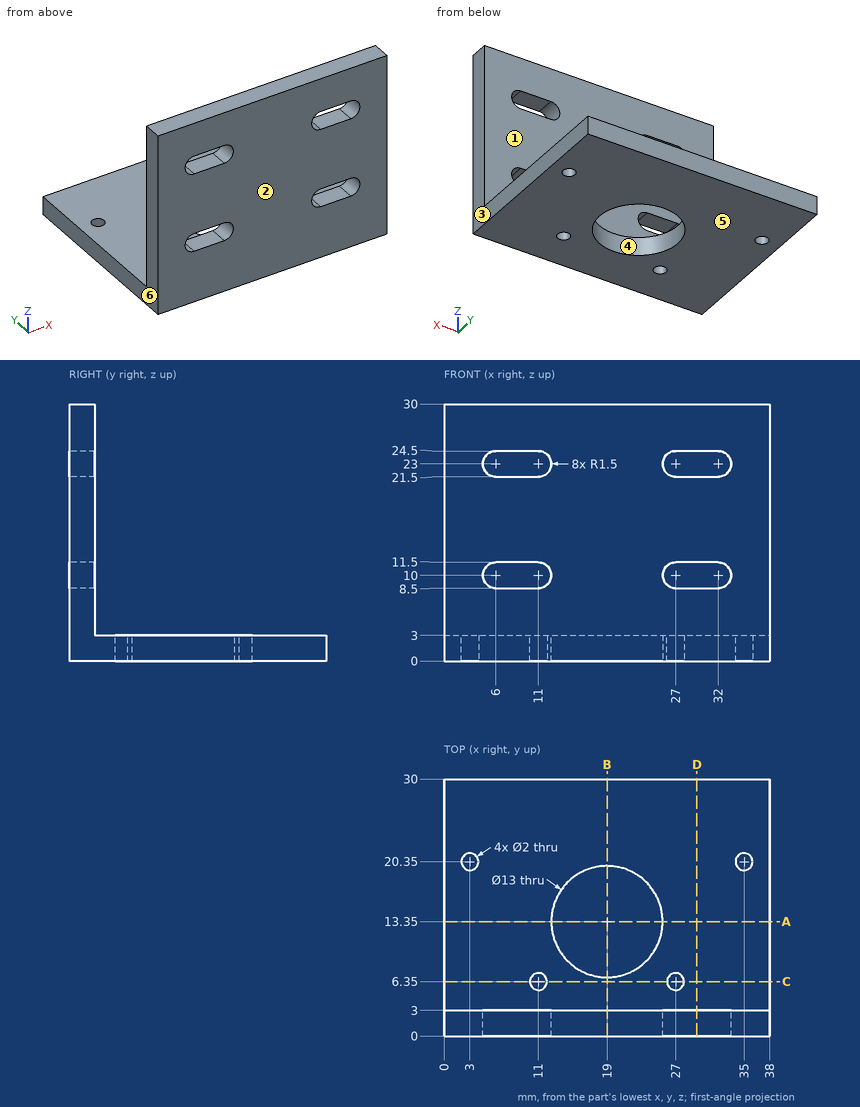
Geometry check sheet. Reference: drawing and pictorial views, mm from the part's lowest x, y, z. A direction names the side the tool comes from. Coordinates: 2 decimals unless noted, no trailing zeros. Loops run counter-clockwise (first coordinate to the right, second up) from the corner with the lowest first, then second, coordinate; pieces in that order, holes last.
1) Sectioned sample at D-D (x = 29.5). Record the boundary of the cut face in (y, z).
2) Access from +Z, -Z, +X, -X, +Y, -Y to the whole of each face (thin tool, end or side, straight path). Record for the marked faces 1 and 2.
3) Material ranges on probe 1 along Y at (x, z) = (11, 1.3); probe 2 along Y at (x, z) = (21.5, 1.5); probe 3 along Z at (x, y) = (35, 23.5), recorded low to high.
4) Sectioned sample at A-A (y = 13.35). Record the boundary of the cut face in (x, z), and give its area (3 significant figures).
5) Gauge pin test, flat ends, axial feed: pin 1 (2.5 mm diameter, centred on x = 35, y = 20.35, fed in from +Z); pin 2 (6 mm diameter, centred on x = 11.5, z = 21, fed in from +Y). Record the tip position at first contact, or that the pin passes through.
6) Release check for a two-part mould opening along X. For the marked faces 3, 4, 5 and 6 record: released by +X, released by -X, zero draft, split by the parting line, or undercut.
7) Sectioned sample at B-B (x = 19). Record the boundary of the cut face in (y, z).
8) Sectioned sample at C-C (y = 6.35). Record the boundary of the cut face in (x, z), and give its area (3 significant figures).
Check sheet entries:
1. outline: (0, 0) - (30, 0) - (30, 3) - (3, 3) - (3, 8.5) - (0, 8.5) - close; (0, 11.5) - (3, 11.5) - (3, 21.5) - (0, 21.5) - close; (0, 24.5) - (3, 24.5) - (3, 30) - (0, 30) - close
2. face 1: +Z, +X, -X, +Y
2. face 2: +Z, -Z, +X, -X, -Y
3. probe 1: y = 0 to 5.35, 7.35 to 30
3. probe 2: y = 0 to 7.35, 19.35 to 30
3. probe 3: z = 0 to 3
4. outline: (0, 0) - (12.5, 0) - (12.5, 3) - (0, 3) - close; (25.5, 0) - (38, 0) - (38, 3) - (25.5, 3) - close
4. area: 75.0 mm2
5. pin 1: stops at z = 3
5. pin 2: stops at y = 3
6. face 3: released by +X
6. face 4: undercut
6. face 5: zero draft
6. face 6: released by -X
7. outline: (0, 0) - (6.85, 0) - (6.85, 3) - (3, 3) - (3, 30) - (0, 30) - close; (19.85, 0) - (30, 0) - (30, 3) - (19.85, 3) - close
8. outline: (0, 0) - (10, 0) - (10, 3) - (0, 3) - close; (12, 0) - (26, 0) - (26, 3) - (12, 3) - close; (28, 0) - (38, 0) - (38, 3) - (28, 3) - close
8. area: 102 mm2
